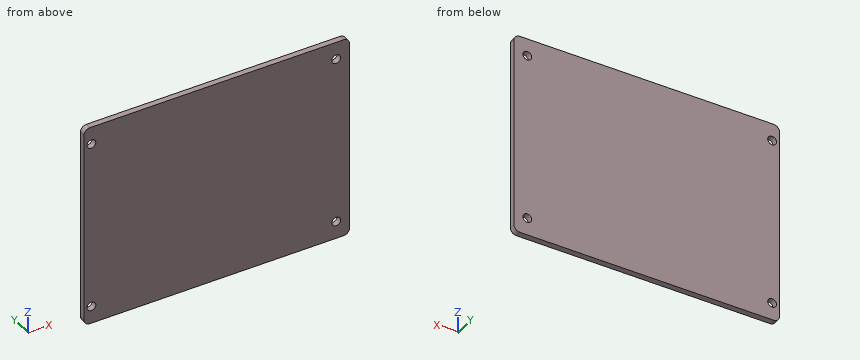
from build123d import *

# Parameters (mm, degrees)
CROQUIS1_W              = 90
CROQUIS1_H              = 70
CROQUIS1_R              = 1.5
SALIENTE_EXTRUIR1_DEPTH = 2
REDONDEO1_R             = 2


with BuildPart() as part:
    # Croquis1 → Saliente-Extruir1 (new body)
    with BuildSketch(Plane(origin=(0, 0, 0), x_dir=(1, 0, 0), z_dir=(0, 1, 0))):
        Rectangle(CROQUIS1_W, CROQUIS1_H)
        with Locations(Location((-42.5, -29, 0), (0, 0, 270))):
            Circle(CROQUIS1_R, mode=Mode.SUBTRACT)
        with Locations(Location((-42.5, 29, 0), (0, 0, 270))):
            Circle(CROQUIS1_R, mode=Mode.SUBTRACT)
        with Locations(Location((40.5, -29, 0), (0, 0, 270))):
            Circle(CROQUIS1_R, mode=Mode.SUBTRACT)
        with Locations(Location((40.5, 29, 0), (0, 0, 270))):
            Circle(CROQUIS1_R, mode=Mode.SUBTRACT)
    extrude(amount=SALIENTE_EXTRUIR1_DEPTH)

    # Redondeo1
    redondeo1_edges = [part.edges().sort_by_distance(p)[0] for p in [
        (-45, 1, -35),
        (45, 1, -35),
        (45, 1, 35),
        (-45, 1, 35),
    ]]
    fillet(redondeo1_edges, radius=REDONDEO1_R)


solid = part.part
The model under review builds one solid part; all positions refer to its coordinate system, in mm. Coordinates: 2 decimals unless noted, no trailing zeros. Loops run counter-clockwise (first coordinate to the right, second up) from the corner with the lowest first, then second, coordinate; pieces in that order, holes last. Notation, with made-up numbers: M 24,46.5 L 71,46.5 A27 ccw 71,81.5 Z; hole C 85.25,64.5 d1. An arc over 180 degrees is marked long. Put each result on its own line as item: value. Start each with the question number.
Q1. Wall thickness on line 1 (X direction, y = 1.25, z = 29): over which ranges is the line inside the solid? List them lowest first.
Q2. Clearance check with a flat-ended pin moving along its axis: pin 1 (2.5 mm diameter, centred on x = -42.5, z = 29, fed in from -Y). State where the tip first meets the part, or that it passes through.
Q3. Add section A-A (z = 29). Write out the cut boundary in (x, y), and give its area (3 significant figures).
Q4. Add section B-B (x = 40.5). Write out the cut boundary in (y, z).
Answers:
1. line 1: x = -45 to -44, -41 to 39, 42 to 45
2. pin 1: passes through
3. outline: M -45,0 L -44,0 L -44,2 L -45,2 Z; M -41,0 L 39,0 L 39,2 L -41,2 Z; M 42,0 L 45,0 L 45,2 L 42,2 Z
3. area: 168 mm^2
4. outline: M 0,-35 L 2,-35 L 2,-30.5 L 0,-30.5 Z; M 0,-27.5 L 2,-27.5 L 2,27.5 L 0,27.5 Z; M 0,30.5 L 2,30.5 L 2,35 L 0,35 Z
